from build123d import *

# Parameters (mm, degrees)
F0_W     = 103.557102
F0_H     = 68.452998
F1_DEPTH = 50
F2_R     = 8.015523
F3_DEPTH = 70
F5_DEPTH = 75
F7_DEPTH = 60
F8_R     = 8.775405
F9_DEPTH = 75
F10_R    = 5


with BuildPart() as f1:
    # F0 (on Front) → F1 (new body)
    with BuildSketch(Plane.XZ):
        Rectangle(F0_W, F0_H)
    extrude(amount=-F1_DEPTH)

    # F2 (on face) → F3 (cut)
    with BuildSketch(Plane.XY.offset(34.226499)):
        with Locations((-27.760793, 25)):
            Circle(F2_R)
    extrude(amount=-F3_DEPTH, mode=Mode.SUBTRACT)

    # F4 (on face) → F5 (cut)
    with BuildSketch(Plane.XY.offset(34.226499)):
        with BuildLine():
            Line((51.778551, 33.015523), (-27.760793, 33.015523))
            ThreePointArc((-27.760793, 33.015523), (-22.092962, 30.667831), (-19.74527, 25))
            ThreePointArc((-19.74527, 25), (-22.042391, 19.383196), (-27.617118, 16.985765))
            Line((-27.617118, 16.985765), (51.778551, 18.409128))
            Line((51.778551, 18.409128), (51.778551, 33.015523))
        make_face()
    extrude(amount=-F5_DEPTH, mode=Mode.SUBTRACT)

    # F6 (on face) → F7 (cut)
    with BuildSketch(Plane.XZ):
        Polygon((51.778551, 34.226499), (23.059108, 34.226499), (51.778551, 0), align=None)
    extrude(amount=-F7_DEPTH, mode=Mode.SUBTRACT)

    # F8 (on face) → F9 (cut)
    with BuildSketch(Plane.XZ):
        with Locations((27.760791, -17.11325)):
            Circle(F8_R)
    extrude(amount=-F9_DEPTH, mode=Mode.SUBTRACT)

    # F10
    f10_edges = [f1.edges().sort_by_distance(p)[0] for p in [
        (-51.778551, 0, 0),
        (-51.778551, 50, 0),
    ]]
    fillet(f10_edges, radius=F10_R)


solid = f1.part
Verification items for the finished model (mm, model axes). Round coordinates to 2 decimals unless told otherwise and drop trailing zeros. Order: outer loops, then holes, each group sorted by start corner. A loop starts at its lowest first (then second) coordinate and runs counter-clockwise, first axis right, second up.
1. Thickness scan on L1, parallel to Y at x = 2, z = 22; L2, parallel to Y at x = 19, z = 9.5; L3, parallel to X at y = 13, z = -10.5. Record the ranges inside material, lowest first.
Final values:
L1: y = 0 to 17.52, 33.02 to 50
L2: y = 0 to 17.82, 33.02 to 50
L3: x = -51.78 to 21.99, 33.53 to 51.78
2. Section check C-C on y = 25. Record the cut outline in (x, z).
Final values:
outline: (-51.78, -34.23) - (-35.78, -34.23) - (-35.78, 34.23) - (-51.78, 34.23) - close
3. Go/stop test with flat-tipped pins: P1, Ø16, axis at x = 27.76, z = -17.11, coming from the -Y side; P2, Ø6, axis at x = 30.5, y = 39.5, coming from the +Z side. Record where each tip stops, or that it passes through.
Final values:
P1: passes through
P2: stops at z = 28.93
4. Section check A-A on x = -24. Record the cut outline in (y, z), then the cut area to 3 significant figures.
Final values:
outline: (0, -34.23) - (17.05, -34.23) - (17.05, 34.23) - (0, 34.23) - close; (33.02, -34.23) - (50, -34.23) - (50, 34.23) - (33.02, 34.23) - close
area: 2,330 mm2
5. Section check B-B on z = -14.5. Record the cut outline in (x, y), then the cut area to 3 significant figures.
Final values:
outline: (-51.78, 5) arc R5 ccw to (-46.78, 0) - (19.38, 0) - (19.38, 17.83) - (-27.62, 16.99) arc R8.02 cw (long way) to (-27.76, 33.02) - (19.38, 33.02) - (19.38, 50) - (-46.78, 50) arc R5 ccw to (-51.78, 45) - close; (36.14, 0) - (51.78, 0) - (51.78, 18.41) - (36.14, 18.13) - close; (36.14, 33.02) - (51.78, 33.02) - (51.78, 50) - (36.14, 50) - close
area: 3,260 mm2
6. Release check for a two-part mould opening along Y. For faces 1 (the cylindrical face through (20.797, 8.941, -22.453)), 2 (the cylindrical face through (-50.35, 48.5, 0.48)), 3 (the flat face through (13, 33.016, 0)), 4 (the cylindrical face through (-35.776, 25.105, 0.479)) record: +Y half, -Y half, draft (parallel to the pull), parting line (faces both ways), or undercut.
Final values:
face 1: draft
face 2: +Y half
face 3: undercut
face 4: undercut
7. Section check D-D on y = 14. Record the cut outline in (x, z), then the cut area to 3 significant figures.
Final values:
outline: (-51.78, -34.23) - (51.78, -34.23) - (51.78, 0) - (23.06, 34.23) - (-51.78, 34.23) - close; hole circle Ø17.55 at (27.76, -17.11)
area: 6,360 mm2
